Part print with two shaded views. Sizes in mm from the minimum x, y, z corner. A direction names the side the tool comes from. Give positions to 0.01 mm unless a question says otherwise; leave off trailing zeros. Write each loop counter-clockwise with the first axis right and the second up, starting at its lowest first coordinate (ties: lowest second). Pieces come first, ordered by that corner, then holes. Notation, with made-up numbers: (60, 44) - (84, 44) arc R26 ccw to (84, 60) - close; hole circle Ø2 at (44.25, 20). An arc over 180 degrees is marked (long way). Answer as a JSON object with one key per item and string values.
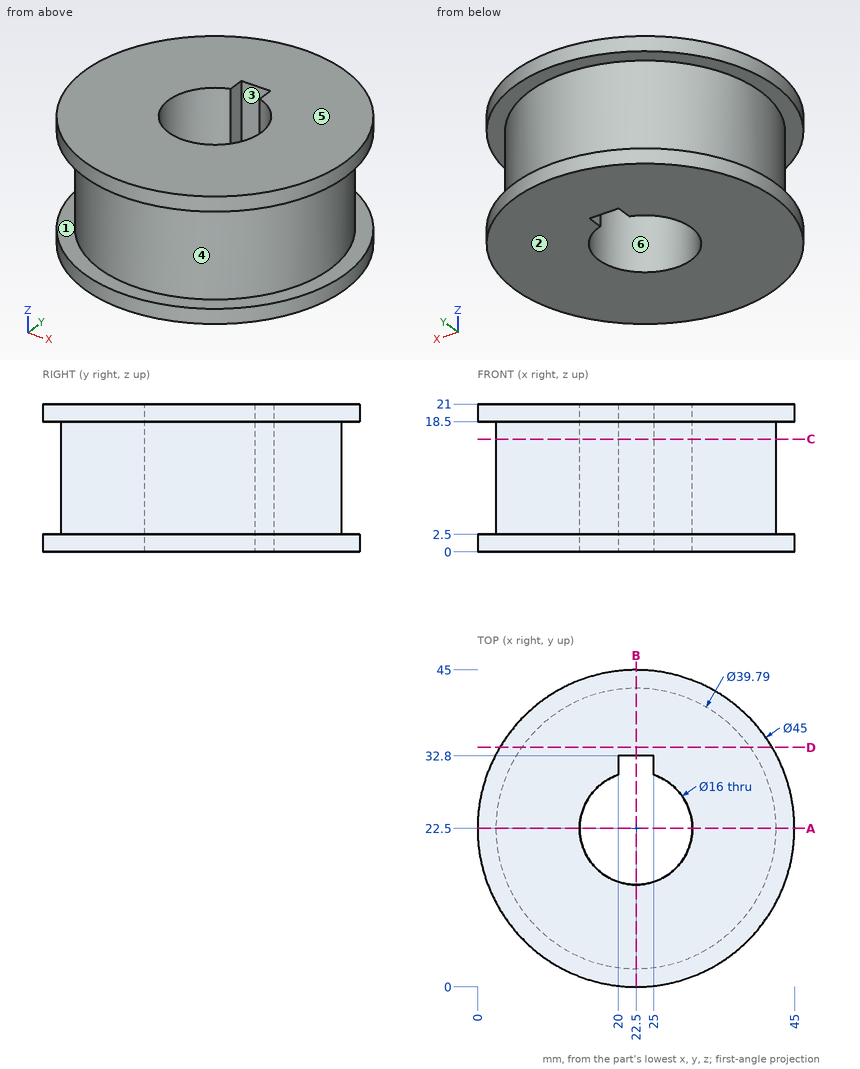
(1) Pull direction X, two halves, no side cores. Call the marked faces 3, 4, 5 and 6: pulls with the +X half, pulls with the -X half, needs draft (parallel to the pull), parting line crosses it, or undercut.
Answer key:
{"face 3": "undercut", "face 4": "parting line crosses it", "face 5": "needs draft", "face 6": "undercut"}
(2) Saw through at D-D, the plane y = 34. Give the cut face in (x, z).
Answer key:
{"outline": "(3.16, 0) - (41.84, 0) - (41.84, 2.5) - (38.73, 2.5) - (38.73, 18.5) - (41.84, 18.5) - (41.84, 21) - (3.16, 21) - (3.16, 18.5) - (6.27, 18.5) - (6.27, 2.5) - (3.16, 2.5) - close"}
(3) Flat gauge pins, fed straight in: P1, Ø2.5, axis at x = 22, z = 12.5, coming from the -Y side (3 decimals); P2, Ø12, axis at y = 36, z = 10.5, coming from the -X side; P3, Ø6, axis at y = 14, z = 3.5, coming from the +X side. Where does each tip first touch, or does it go through?
Answer key:
{"P1": "stops at y = 2.605", "P2": "stops at x = 4.07", "P3": "stops at x = 44.27"}
(4) Saw through at A-A, the plane y = 22.5. Give the cut face in (x, z) (3 decimals).
Answer key:
{"outline": "(0, 0) - (14.5, 0) - (14.5, 21) - (0, 21) - (0, 18.5) - (2.605, 18.5) - (2.605, 2.5) - (0, 2.5) - close; (30.5, 0) - (45, 0) - (45, 2.5) - (42.395, 2.5) - (42.395, 18.5) - (45, 18.5) - (45, 21) - (30.5, 21) - close"}
(5) 3-axis set-ups, long thin cutter, end or side, ignore diameter. For the marked faces 1 and 2: which of +Z, -Z, +X, -X, +Y, -Y reach the whole face in a straight line?
Answer key:
{"face 1": "none", "face 2": "-Z, +X, -X, +Y, -Y"}
(6) Saw through at B-B, the plane x = 22.5. Give the cut face in (y, z) (3 decimals), and give its area (3 significant figures).
Answer key:
{"outline": "(0, 0) - (14.5, 0) - (14.5, 21) - (0, 21) - (0, 18.5) - (2.605, 18.5) - (2.605, 2.5) - (0, 2.5) - close; (32.8, 0) - (45, 0) - (45, 2.5) - (42.395, 2.5) - (42.395, 18.5) - (45, 18.5) - (45, 21) - (32.8, 21) - close", "area": "477 mm²"}
(7) Probe L1, parallel to Z at x = 22.5, y = 42.5; L2, parallel to Y at x = 22.5, z = 8.5 (3 decimals); L3, parallel to X at y = 17, z = 6. List the from-to ranges inside material, lowest first. Write a range as [from, to].
Answer key:
{"L1": "z = [0, 2.5], [18.5, 21]", "L2": "y = [2.605, 14.5], [32.8, 42.395]", "L3": "x = [3.38, 16.69], [28.31, 41.62]"}
(8) Saw through at C-C, the plane z = 16. Give the cut face in (x, y) (3 decimals), and give its area (3 significant figures).
Answer key:
{"outline": "circle Ø39.79 at (22.5, 22.5); hole (20, 30.099) arc R8 ccw (long way) to (25, 30.099) - (25, 32.8) - (20, 32.8) - close", "area": "1,030 mm²"}
